```python
from build123d import *

# Parameters (mm, degrees)
F0_W          = 38.1
F0_H          = 44.45
F1_DEPTH      = 10.16
F3_DEPTH      = 6.35
F6_DEPTH      = 3.175
F6_DEPTH_BACK = 3.175
F8_DEPTH      = 7.62
F9_W          = 5.08
F9_H          = 5.08
F10_DEPTH     = 7.62


with BuildPart() as f1:
    # F0 (on Top) → F1 (new body)
    with BuildSketch(Plane.XY):
        Rectangle(F0_W, F0_H)
    extrude(amount=F1_DEPTH)

    # F2 (on face) → F3 (cut)
    with BuildSketch(Plane.XY.offset(10.16)):
        Polygon((14.6646968374, 6.35), (7.3323484187, 19.05), (-7.3323484187, 19.05), (-14.6646968374, 6.35), (-7.3323484187, -6.35), (7.3323484187, -6.35), align=None)
    extrude(amount=-F3_DEPTH, mode=Mode.SUBTRACT)

    # F5 (on offset) → F6 (cut, two sides)
    with BuildSketch(Plane.XZ.offset(15.24)) as f6_sk:
        Polygon((7.3645809335, 3.8287173206), (14.6646495373, 16.547299463), (7.3000686039, 29.2286353945), (-7.3645809335, 29.1913891837), (-14.6646495373, 16.4728070413), (-7.3000686039, 3.7914711098), align=None)
    extrude(amount=-F6_DEPTH, mode=Mode.SUBTRACT)
    extrude(f6_sk.sketch, amount=F6_DEPTH_BACK, mode=Mode.SUBTRACT)

    # F7 (on face) → F8 (cut)
    with BuildSketch(Plane.XY.offset(10.16)):
        Polygon((-10.644121265, -6.985), (-12.1105909488, -4.445), (-15.0435303163, -4.445), (-16.51, -6.985), (-15.0435303163, -9.525), (-12.1105909488, -9.525), align=None)
    extrude(amount=-F8_DEPTH, mode=Mode.SUBTRACT)

    # F9 (on face) → F10 (cut)
    with BuildSketch(Plane.XY.offset(10.16)):
        with Locations((13.97, -6.985)):
            Rectangle(F9_W, F9_H)
    extrude(amount=-F10_DEPTH, mode=Mode.SUBTRACT)


solid = f1.part
```
Work out the finished part from the listing and answer in its coordinate system (mm). Round coordinates to 2 decimals unless told otherwise and drop trailing zeros. Write each loop counter-clockwise with the first axis right and the second up, starting at its lowest first coordinate (ties: lowest second). Pieces come first, ordered by that corner, then holes.
1) Consider probe 1 along Y at (x, z) = (-7, 4.25) (3 decimals); probe 2 along Y at (x, z) = (8, 5) (3 decimals); probe 3 along X at (y, z) = (-9, 3.5). Determine where each line is inside the solid, lowest interval first.
2) Determine the mould class of faces 1 (the face through (0, -22.225, 5)), 2 (the face through (-11, 0, 7)), 3 (the face through (-19.05, 0, 5)) for opening direction Y: pulls with the +Y half, pulls with the -Y half, needs draft (parallel to the pull), parting line crosses it, or undercut.
3) A cutting plane is placed at B-B on x = -16. Determine the outline of the cut face in (y, z) (3 decimals), and give its area (3 significant figures).
4) A cutting plane is placed at A-A on y = -16. Determine the outline of the cut face in (x, z), and give its area (3 significant figures).
5) A cutting plane is placed at C-C on z = 8. Determine the outline of the cut face in (x, y) (3 decimals).
6) A flat-ended cylindrical pin translates along its axis: P1, Ø4, axis at x = -14.5, y = -7.5, coming from the +Z side. Find the tip coordinate at first contact, or state that the pin passes through.
Entries:
1. probe 1: y = -22.225 to -18.415, -12.065 to -6.35, 19.05 to 22.225
1. probe 2: y = -22.225 to -18.415, -12.065 to -5.194, 17.894 to 22.225
1. probe 3: x = -19.05 to -15.35, -11.81 to 11.43, 16.51 to 19.05
2. face 1: pulls with the -Y half
2. face 2: undercut
2. face 3: needs draft
3. outline: (-22.225, 0) - (22.225, 0) - (22.225, 10.16) - (-6.102, 10.16) - (-6.102, 2.54) - (-7.868, 2.54) - (-7.868, 10.16) - (-22.225, 10.16) - close
3. area: 438 mm2
4. outline: (-19.05, 0) - (19.05, 0) - (19.05, 10.16) - (11, 10.16) - (7.36, 3.83) - (-7.3, 3.79) - (-11, 10.16) - (-19.05, 10.16) - close
4. area: 271 mm2
5. outline: (-19.05, -22.225) - (19.05, -22.225) - (19.05, 22.225) - (-19.05, 22.225) - close; hole (-16.51, -6.985) - (-15.044, -9.525) - (-12.111, -9.525) - (-10.644, -6.985) - (-12.111, -4.445) - (-15.044, -4.445) - close; hole (-14.665, 6.35) - (-7.332, -6.35) - (7.332, -6.35) - (14.665, 6.35) - (7.332, 19.05) - (-7.332, 19.05) - close; hole (-9.744, -18.415) - (9.759, -18.415) - (9.759, -12.065) - (-9.744, -12.065) - close; hole (11.43, -9.525) - (16.51, -9.525) - (16.51, -4.445) - (11.43, -4.445) - close
6. P1: stops at z = 10.16
